```python
from build123d import *

# Parameters (mm, degrees)
SKETCH1_W           = 40
SKETCH1_H           = 20
SKETCH1_R           = 2
SKETCH1_R_2         = 2.5
BOSS_EXTRUDE1_DEPTH = 5
CHAMFER1_SIZE       = 1
CUT_EXTRUDE1_DEPTH  = 4
FILLET1_R           = 2


with BuildPart() as part:
    # Sketch1 → Boss-Extrude1 (new, symmetric)
    with BuildSketch(Plane(origin=(0, 0, 0), x_dir=(1, 0, 0), z_dir=(0, 1, 0))):
        Rectangle(SKETCH1_W, SKETCH1_H)
        with Locations(Location((-16, 6, 0), (0, 0, 270))):
            Circle(SKETCH1_R, mode=Mode.SUBTRACT)
        with Locations(Location((16, 6, 0), (0, 0, 270))):
            Circle(SKETCH1_R, mode=Mode.SUBTRACT)
        with Locations(Location((16, -6, 0), (0, 0, 270))):
            Circle(SKETCH1_R, mode=Mode.SUBTRACT)
        with Locations(Location((-16, -6, 0), (0, 0, 270))):
            Circle(SKETCH1_R, mode=Mode.SUBTRACT)
        with Locations(Location((0, 0, 0), (0, 0, 270))):
            Circle(SKETCH1_R_2, mode=Mode.SUBTRACT)
    extrude(amount=BOSS_EXTRUDE1_DEPTH, both=True)

    # Sketch2 → Cut-Revolve1 (revolve, cut)
    with BuildSketch(Plane.XY):
        with BuildLine():
            Line((-12.5, 5), (12.5, 5))
            ThreePointArc((12.5, 5), (11.035533906, 1.464466094), (7.5, 0))
            Line((7.5, 0), (-7.5, 0))
            ThreePointArc((-7.5, 0), (-11.035533906, 1.464466094), (-12.5, 5))
        make_face()
    revolve(axis=Axis((-12.5, 5, 0), (1, 0, 0)), mode=Mode.SUBTRACT)

    # Chamfer1
    chamfer1_edges = [part.edges().sort_by_distance(p)[0] for p in [
        (-16, -5, -8),
        (16, -5, -8),
        (16, -5, 4),
        (-16, -5, 4),
    ]]
    chamfer(chamfer1_edges, length=CHAMFER1_SIZE)

    # Sketch3 → Cut-Extrude1 (cut)
    with BuildSketch(Plane.XZ.offset(5)):
        with BuildLine():
            Line((-5.607695155, 7), (5.607695155, 7))
            ThreePointArc((5.607695155, 7), (12.607695155, 0), (5.607695155, -7))
            Line((5.607695155, -7), (-5.607695155, -7))
            ThreePointArc((-5.607695155, -7), (-12.607695155, 0), (-5.607695155, 7))
        make_face()
    extrude(amount=-CUT_EXTRUDE1_DEPTH, mode=Mode.SUBTRACT)

    # Fillet1
    fillet1_edges = [part.edges().sort_by_distance(p)[0] for p in [
        (-12.607695155, -1, 0),
        (0, -1, 7),
        (12.607695155, -1, 0),
        (0, -1, -7),
    ]]
    fillet(fillet1_edges, radius=FILLET1_R)


solid = part.part
```
Verification items for the finished model (mm, model axes). A direction names the side the tool comes from. Coordinates: 2 decimals unless noted, no trailing zeros. Order: outer loops, then holes, each group sorted by start corner. A loop starts at its lowest first (then second) coordinate and runs counter-clockwise, first axis right, second up. Notation, with made-up numbers: (75, -40) -> (109, -40) arc R26 cw to (109, -23) -> close; hole circle Ø2 at (-20.75, -38). An arc over 180 degrees is marked (long way). Answer as CSV lines item,"result". Start each with the question number.
1) Material ranges on L1, parallel to X at y = 1, z = 6; L2, parallel to Z at x = 17.5, y = -4.5; L3, parallel to X at y = -2.5, z = -4.25, recorded low to high. Write a range as [from, to].
2) Cross-section at D-D, the plane z = -6. Give the number of separate pieces and of enclosed holes in the cut face, then the cut area to 3 significant figures.
3) Cross-section at C-C, the plane y = -4.5. Record the boundary of the cut face in (x, z).
4) Cross-section at B-B, the plane x = 0. Record the boundary of the cut face in (y, z).
5) Set-up check for faces 1 (the face through (0, -4, -7)), 2 (the face through (18, 0, -6)): record each of +Z, -Z, +X, -X, +Y, -Y from which the full face is reachable in a straight line by a thin tool's end or side.
6) Gauge pin test, flat ends, axial feed: pin 1 Ø1 at (x, z) = (-10.5, 0) entering from +Y; pin 2 Ø8 at (x, z) = (-1, 2.5) entering from -Y; pin 3 Ø4.5 at (x, z) = (-16, 6) entering from -Y. Record the tip position at first contact, or that the pin passes through.
7) Cross-section at A-A, the plane z = 0. Record the boundary of the cut face in (x, y), then the cut area to 3 significant figures.
8) Release check for a two-part mould opening along Z. For faces 3 (the face through (0, 0, -10)), 4 (the face through (0, 1, 3)), 5 (the face through (-20, 0, 0)) record: released by +Z, released by -Z, zero draft, split by the parting line, or undercut.
Conclusion:
1,L1,"x = [-20, -18], [-14, 14], [18, 20]"
1,L2,"z = [-10, -8], [-4, 4], [8, 10]"
1,L3,"x = [-20, -16.97], [-15.03, -11.09], [11.09, 15.03], [16.97, 20]"
2,separate pieces,"3"
2,enclosed holes,"0"
2,area,"252 mm²"
3,outline,"(-20, -10) -> (20, -10) -> (20, 10) -> (-20, 10) -> close; hole circle Ø5 at (-16, -6); hole circle Ø5 at (-16, 6); hole (-5.61, -7) -> (5.61, -7) arc R7 ccw to (5.61, 7) -> (-5.61, 7) arc R7 ccw to start; hole circle Ø5 at (16, -6); hole circle Ø5 at (16, 6)"
4,outline,"(-5, -10) -> (5, -10) -> (5, -5) arc R5 cw to (0.67, -2.5) -> (-1, -2.5) -> (-1, -5) arc R2 cw to (-3, -7) -> (-5, -7) -> close; (-5, 7) -> (-3, 7) arc R2 cw to (-1, 5) -> (-1, 2.5) -> (0.67, 2.5) arc R5 cw to (5, 5) -> (5, 10) -> (-5, 10) -> close"
5,face 1,"-Y"
5,face 2,"+Y, -Y"
6,pin 1,"stops at y = 1.43"
6,pin 2,"stops at y = -1.68"
6,pin 3,"stops at y = -4.25"
7,outline,"(-20, -5) -> (-12.61, -5) -> (-12.61, -3) arc R2 cw to (-10.61, -1) -> (-2.5, -1) -> (-2.5, 0) -> (-7.5, 0) arc R5 cw to (-12.5, 5) -> (-20, 5) -> close; (2.5, -1) -> (10.61, -1) arc R2 cw to (12.61, -3) -> (12.61, -5) -> (20, -5) -> (20, 5) -> (12.5, 5) arc R5 cw to (7.5, 0) -> (2.5, 0) -> close"
7,area,"182 mm²"
8,face 3,"released by -Z"
8,face 4,"undercut"
8,face 5,"zero draft"
